CAD build for the part. Positions are in the model's coordinates, mm. A direction names the side the tool comes from. Round coordinates to 2 decimals unless told otherwise and drop trailing zeros. Loops run counter-clockwise (first coordinate to the right, second up) from the corner with the lowest first, then second, coordinate; pieces in that order, holes last.
Autodesk Inventor part; units mm, degrees
ref_plane "YZ Plane" through (0, 0, 0) normal (1, 0, 0) x (0, 1, 0)
ref_plane "XZ Plane" through (0, 0, 0) normal (0, 1, 0) x (-1, 0, 0)
ref_plane "XY Plane" through (0, 0, 0) normal (0, 0, 1) x (1, 0, 0)
sketch "Sketch1" plane through (0, 0, 0) normal (0, 1, 0) x (-1, 0, 0)
  arc A0 (14.6882, 29.8139) -> (14.6882, 33.0139) centre (14.6882, 31.4139) ccw
  circle A1 centre (14.6882, 7.9139) radius 1.6
  line L0 (14.6882, -2.0861) -> (8.1882, -2.0861)
  arc A2 (14.6882, 29.8139) -> (3.7382, 26.8799) centre (14.6882, 7.9139) ccw
  arc A3 (14.6882, 33.0139) -> (2.1382, 29.6511) centre (14.6882, 7.9139) ccw
  arc A4 (14.6882, 37.9139) -> (-0.3118, 33.8947) centre (14.6882, 7.9139) ccw
  line L1 (24.6882, -2.0861) -> (24.6882, -5.0861)
  line L2 (24.6882, -5.0861) -> (14.6882, -5.0861)
  line L3 (14.6882, -5.0861) -> (14.6882, -2.0861)
  line L4 (8.1846, 14.2314) -> (8.1882, -2.0861)
  line L5 (39.6882, -2.0861) -> (24.6882, -2.0861)
  line L6 (49.6882, -2.0861) -> (49.6882, -5.0861)
  line L7 (49.6882, -5.0861) -> (39.6882, -5.0861)
  line L8 (39.6882, -5.0861) -> (39.6882, -2.0861)
  line L9 (49.6882, -2.0861) -> (54.6882, -2.0861)
  arc A5 (2.1382, 29.6511) -> (3.7382, 26.8799) centre (2.9382, 28.2655) ccw
  arc A6 (-0.3118, 33.8947) -> (2.9382, 21.7655) centre (2.9382, 28.2655) ccw
  line L10 (8.1846, 14.2314) -> (8.1846, 16.7655)
  arc A7 (8.1846, 16.7655) -> (3.1846, 21.7655) centre (3.1846, 16.7655) ccw
  line L11 (3.1846, 21.7655) -> (2.9382, 21.7655)
  arc A8 (19.2844, 36.0101) -> (14.6882, 37.9139) centre (14.6882, 31.4139) ccw
  line L12 (54.6882, -2.0861) -> (54.6882, 5.4139)
  arc A9 (54.6882, 5.4139) -> (47.6724, 12.8983) centre (47.1882, 5.4139) ccw
  arc A10 (38.0341, 17.2604) -> (47.6724, 12.8983) centre (48.6407, 27.867) ccw
  line L13 (19.2844, 36.0101) -> (38.0341, 17.2604)
extrude "Extrusion1" add sketch "Sketch1" along normal blind 3
properties part number "camMount"
Item 1: 3-axis set-ups, long thin cutter, end or side, ignore diameter. For faces 4 (the cylindrical face through (-16.288, 1.479, 31.449)), 5 (the flat face through (-49.688, 1, -4)), 6 (the flat face through (-32, 1, -2.086)): which of +Z, -Z, +X, -X, +Y, -Y reach the whole face in a straight line?
Answers follow:
face 4: +Y, -Y
face 5: -Z, -X, +Y, -Y
face 6: -Z, +Y, -Y
Item 2: Two-plate mould, pull along Z, no slides. Class faces 1 (the cylindrical face through (-42.525, 1.479, 14.17)), 2 (the flat face through (-39.688, 1, -4)), 3 (the cylindrical face through (-8.103, 1.479, 32.135)): released by +Z, released by -Z, zero draft, split by the parting line, or undercut.
Answers follow:
face 1: released by +Z
face 2: zero draft
face 3: undercut
Item 3: Cut at C-C, the plane y = 1. Give the cut face in (x, z), plus the area to 3 significant figures.
Answers follow:
outline: (-54.69, -2.09) - (-49.69, -2.09) - (-49.69, -5.09) - (-39.69, -5.09) - (-39.69, -2.09) - (-24.69, -2.09) - (-24.69, -5.09) - (-14.69, -5.09) - (-14.69, -2.09) - (-8.19, -2.09) - (-8.18, 14.23) - (-8.18, 16.77) arc R5 cw to (-3.18, 21.77) - (-2.94, 21.77) arc R6.5 ccw to (0.31, 33.89) arc R30 ccw to (-14.69, 37.91) arc R6.5 ccw to (-19.28, 36.01) - (-38.03, 17.26) arc R15 cw to (-47.67, 12.9) arc R7.5 ccw to (-54.69, 5.41) - close; hole circle Ø3.2 at (-14.69, 7.91); hole (-14.69, 29.81) arc R21.9 cw to (-3.74, 26.88) arc R1.6 ccw to (-2.14, 29.65) arc R25.1 ccw to (-14.69, 33.01) arc R1.6 ccw to start
area: 1,380 mm2
Item 4: Flat gauge pins, fed straight in: P1, Ø1.5, axis at x = -40, y = 2, coming from the +Z side; P2, Ø2.5, axis at x = -14.69, z = 7.91, coming from the -Y side; P3, Ø6, axis at x = -7.5, z = 6.5, coming from the -Y side; P4, Ø1.5, axis at x = -52, y = 1.5, coming from the -Z side. Where does each tip first touch, or does it go through?
Answers follow:
P1: stops at z = 16.17
P2: passes through
P3: stops at y = 0
P4: stops at z = -2.09
Item 5: Cut at D-D, the plane z = 29. Give the cut face in (x, y), plus the area to 3 significant figures.
Answers follow:
outline: (-26.29, 0) - (-8.77, 0) - (-8.77, 3) - (-26.29, 3) - close; (-1.52, 0) - (3.52, 0) - (3.52, 3) - (-1.52, 3) - close
area: 67.7 mm2
Item 6: Cut at A-A, the plane z = 7. Give the cut face in (x, y).
Answers follow:
outline: (-54.52, 0) - (-16, 0) - (-16, 3) - (-54.52, 3) - close; (-13.37, 0) - (-8.19, 0) - (-8.19, 3) - (-13.37, 3) - close
Item 7: Probe line 1 (X direction, y = 1.95, z = 7.5); line 2 (X direction, y = 1.3, z = 8); line 3 (X direction, y = 0.45, z = 5). List the from-to ranges inside material, lowest first.
Answers follow:
line 1: x = -54.39 to -16.23, -13.14 to -8.19
line 2: x = -54.23 to -16.29, -13.09 to -8.19
line 3: x = -54.69 to -8.19
Item 8: Cut at B-B, the plane x = -14. Give the cut face in (y, z).
Answers follow:
outline: (0, -2.09) - (3, -2.09) - (3, 6.47) - (0, 6.47) - close; (0, 9.36) - (3, 9.36) - (3, 29.8) - (0, 29.8) - close; (0, 33) - (3, 33) - (3, 37.91) - (0, 37.91) - close
